Source: three-view drawing plus pictorial views. Frame: mm from the lowest corner of the part. Coordinates: 2 decimals unless noted, no trailing zeros. Order: outer loops, then holes, each group sorted by start corner. A loop starts at its lowest first (then second) coordinate and runs counter-clockwise, first axis right, second up. Notation, with made-up numbers: (37.25, -37.75) - (67.25, -37.75) arc R23 ccw to (67.25, -6.75) - close; hole circle Ø5 at (41.25, 21). An arc over 180 degrees is marked (long way). One line per question, with ' | ' between items.
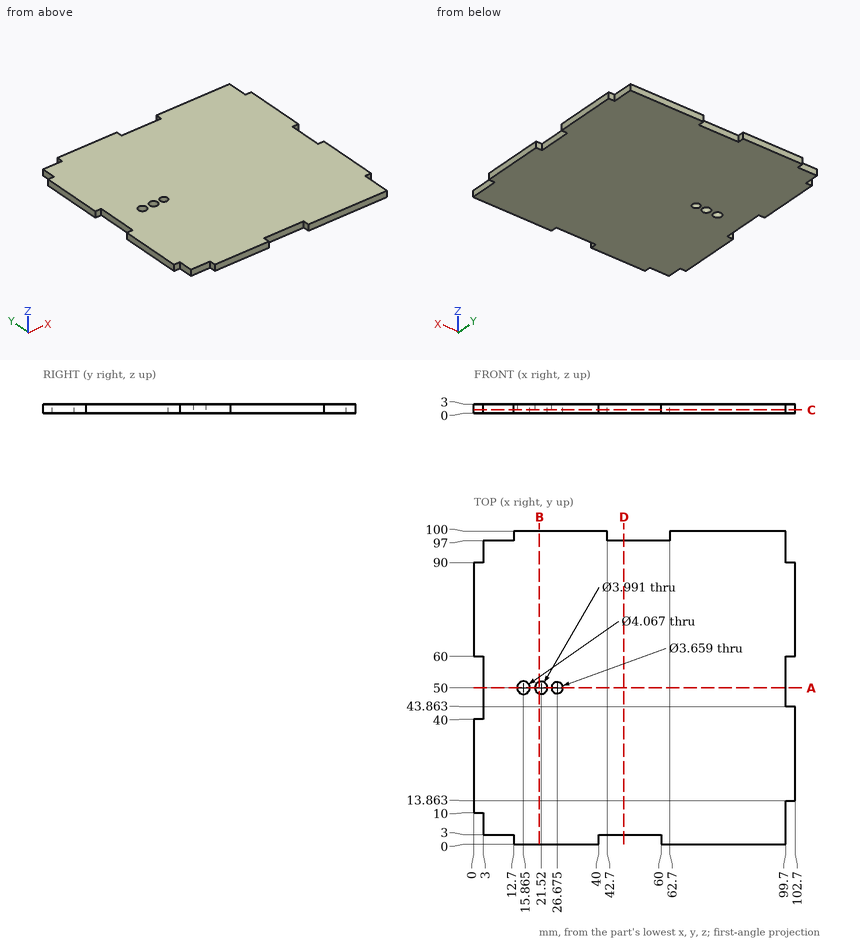
Item 1: Section D-D on x = 48. Return the cut outline in (y, z).
Data:
outline: (3, 0) - (97, 0) - (97, 3) - (3, 3) - close
Item 2: Contact query for flat-ended pins moving along their axis: P1, Ø1.5, axis at y = 6, z = 2, coming from the -X side; P2, Ø2, axis at x = 26.675, y = 50, coming from the -Z side; P3, Ø0.9, axis at x = 2, z = 2, coming from the +Y side; P4, Ø0.9, axis at x = 6, z = 1.5, coming from the +Y side. Output: stop coordinate, or through.
Data:
P1: x = 3 | P2: through | P3: y = 90 | P4: y = 97
Item 3: Section C-C on z = 1.15. Count the separate pieces of the cut face and the enclosed holes in it, and give its area (3 significant figures).
Data:
separate pieces: 1 | enclosed holes: 3 | area: 9,820 mm^2
Item 4: Ray query, line 1 (X direction, y = 13, z = 0.65); line 2 (Y direction, x = 46.5, z = 0.3); line 3 (Y direction, x = 20.5, z = 0.2) (1 decimal). Return the intervals inside material, ascending.
Data:
line 1: 0 to 99.7 | line 2: 3 to 97 | line 3: 0 to 48.3, 51.7 to 100
Item 5: Section B-B on x = 21. Return the cut outline in (y, z).
Data:
outline: (0, 0) - (48.07, 0) - (48.07, 3) - (0, 3) - close; (51.93, 0) - (100, 0) - (100, 3) - (51.93, 3) - close
Item 6: Section A-A on y = 50. Return the cut outline in (x, z) (1 decimal).
Data:
outline: (3, 0) - (13.8, 0) - (13.8, 3) - (3, 3) - close; (17.9, 0) - (19.5, 0) - (19.5, 3) - (17.9, 3) - close; (23.5, 0) - (24.8, 0) - (24.8, 3) - (23.5, 3) - close; (28.5, 0) - (99.7, 0) - (99.7, 3) - (28.5, 3) - close
